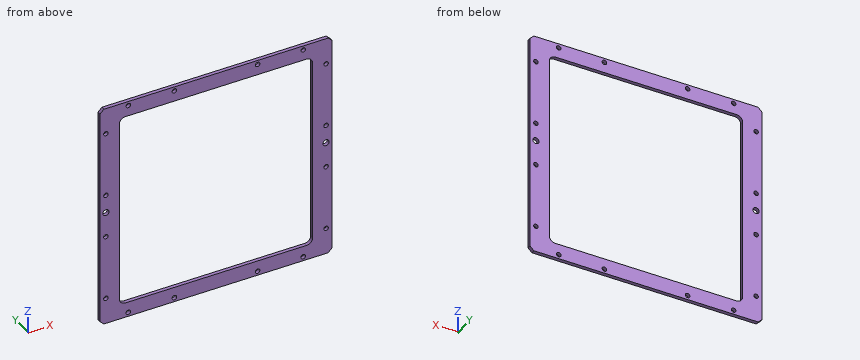
Autodesk Fusion 360 part; units mm, degrees
sketch "Front" plane through (0, 0, 0) normal (0, 1, 0) x (1, 0, 0) in component "1006350A"
  line L0 (-97.5923, -201.9946) -> (221.2351, -201.9946) construction
  line L1 (-99.947, -6.4146) -> (290.3014, -6.4146) construction
  line L2 (12.4997, 61.7326) -> (12.4997, -271.4585) construction
  line L3 (208.0797, 69.9741) -> (208.0797, -187.16) construction
  line L4 (213.4645, 13.4611) -> (213.4645, -265.3363) construction
  line L5 (7.1149, -256.6239) -> (7.1149, 6.397) construction
  line L6 (-10.9391, -2.6046) -> (257.2621, -2.6046) construction
  line L7 (3.4246, -205.8046) -> (275.1579, -205.8046) construction
  line L8 (196.1925, -231.664) -> (196.1925, 4.0423) construction
  line L9 (200.5105, 72.0933) -> (200.5105, -273.8132) construction
  line L10 (20.3229, -271.4585) -> (20.3229, 19.5833) construction
  line L11 (-9.5263, -26.3536) -> (218.174, -26.3536) construction
  line L12 (-30.2477, -84.6466) -> (216.2902, -84.6466) construction
  line L13 (226.8864, -107.3796) -> (-21.2998, -107.3796) construction
  line L14 (-47.6725, -123.7626) -> (220.7641, -123.7626) construction
  line L15 (-72.1615, -182.0556) -> (219.1158, -182.0556) construction
  line L16 (-7.1716, -192.3426) -> (237.718, -192.3426) construction
  line L17 (24.3869, -243.673) -> (24.3869, 8.2807) construction
  line L18 (187.7982, 11.5773) -> (187.7982, -213.2972) construction
  line L19 (147.2467, 23.5863) -> (147.2467, -210.9425) construction
  line L20 (73.3327, 36.3018) -> (73.3327, -224.8353) construction
  line L21 (32.4133, 51.8428) -> (32.4133, -217.3002) construction
  line L22 (267.4197, -11.8756) -> (2.5805, -11.8756) construction
  line L23 (267.0325, -196.4066) -> (1.4189, -196.4066) construction
  line L24 (1.5972, -16.0666) -> (220.1148, -16.0666) construction
  line L25 (7.1149, -205.8046) -> (213.4645, -205.8046)
  line L26 (213.4645, -205.8046) -> (213.4645, -2.6046)
  line L27 (213.4645, -2.6046) -> (7.1149, -2.6046)
  line L28 (7.1149, -2.6046) -> (7.1149, -205.8046)
  line L29 (24.3869, -192.3426) -> (196.1925, -192.3426)
  line L30 (196.1925, -192.3426) -> (196.1925, -16.0666)
  line L31 (196.1925, -16.0666) -> (24.3869, -16.0666)
  line L32 (24.3869, -16.0666) -> (24.3869, -192.3426)
  point P0 (32.4133, -201.9946)
  point P1 (73.3327, -201.9946)
  point P2 (147.2467, -201.9946)
  point P3 (187.7982, -201.9946)
  point P4 (208.0797, -182.0556)
  point P5 (208.0797, -123.7626)
  point P6 (208.0797, -107.3796)
  point P7 (208.0797, -84.6466)
  point P8 (208.0797, -26.3536)
  point P9 (187.7982, -6.4146)
  point P10 (147.2467, -6.4146)
  point P11 (73.3327, -6.4146)
  point P12 (32.4133, -6.4146)
  point P13 (12.4997, -26.3536)
  point P14 (12.4997, -84.6466)
  point P15 (12.4997, -107.3796)
  point P16 (12.4997, -123.7626)
  point P17 (12.4997, -182.0556)
  dimension "d1" = 195.58
  dimension "d2" = 3.81
  dimension "d3" = 19.939
  dimension "d4" = 78.232
  dimension "d5" = 117.348
  dimension "d6" = 175.641
  dimension "d7" = 100.965
  dimension "d10" = 5.3848
  dimension "d11" = 17.272
  dimension "d12" = 60.833
  dimension "d13" = 134.747
  dimension "d14" = 175.6664
  dimension "d15" = 195.58
  dimension "d16" = 203.2
  dimension "d17" = 184.531
  dimension "d18" = 5.461
  dimension "d19" = 13.462
  dimension "d20" = 189.0776
  dimension "d21" = 206.3496
  dimension "d22" = 13.462
  dimension "d33" = 7.5692
  dimension "d34" = 180.1876
extrude "Extrude1" add sketch "Front" along normal blind 3.175 in component "1006350A"
chamfer "Chamfer1" distance 3.556 angle 45 4 edges at (7.1149, 1.5875, 205.8046) (213.4645, 1.5875, 205.8046) (213.4645, 1.5875, 2.6046) (7.1149, 1.5875, 2.6046) in component "1006350A"
fillet "Fillet1" radius 5.5372 4 edges at (196.1925, 1.5875, 192.3426) (24.3869, 1.5875, 192.3426) (24.3869, 1.5875, 16.0666) (196.1925, 1.5875, 16.0666) in component "1006350A"
hole "Hole1" at (12.4997, 0, 107.3796) at (208.0797, 0, 107.3796) direction (0, 1, 0) diameter 5.5372 end through all in component "1006350A"
hole "Hole2" at (147.2467, 0, 201.9946) at (187.7982, 0, 201.9946) at (208.0797, 0, 182.0556) at (208.0797, 0, 123.7626) at (73.3327, 0, 201.9946) at (32.4133, 0, 201.9946) at (12.4997, 0, 182.0556) at (12.4997, 0, 123.7626) at (12.4997, 0, 84.6466) at (12.4997, 0, 26.3536) at (32.4133, 0, 6.4146) at (73.3327, 0, 6.4146) at (147.2467, 0, 6.4146) at (187.7982, 0, 6.4146) at (208.0797, 0, 26.3536) at (208.0797, 0, 84.6466) direction (0, 1, 0) diameter 4.0894 end through all in component "1006350A"
component "1006350A" placed x (1, 0, 0) y (0, 1, 0) z (0, 0, 1) at (0, 0, 0)
Work out the finished part from the listing and answer in its coordinate system (mm). Give positions to 0.01 mm unless a question says otherwise; leave off trailing zeros. Loops run counter-clockwise (first coordinate to the right, second up) from the corner with the lowest first, then second, coordinate; pieces in that order, holes last. Notation, with made-up numbers: (1, 10.25) - (23, 10.25) arc R30 cw to (23, 43.25) - close; hole circle Ø10 at (64.25, -22). An arc over 180 degrees is marked (long way). Answer in a Markdown table with one row per item.
(1) Section C-C (y = 1.45) is taken. State how many separate pieces and enclosed holes the cut face has, and give its area (3 significant figures).
Results list:
| item | result |
|---|---|
| separate pieces | 1 |
| enclosed holes | 19 |
| area | 11,400 mm² |
(2) Section A-A (z = 164.5) is taken. Give the vertices of the cut face in (x, y) (1 decimal).
Results list:
| item | result |
|---|---|
| outline | (7.1, 0) - (24.4, 0) - (24.4, 3.2) - (7.1, 3.2) - close; (196.2, 0) - (213.5, 0) - (213.5, 3.2) - (196.2, 3.2) - close |
(3) Consider L1, parallel to X at y = 1.8, z = 156; L2, parallel to Z at x = 149.5, y = 1.4; L3, parallel to X at y = 0.8, z = 187.5. Determine where each line is inside the solid, lowest interval first. Write a range as [from, to].
Results list:
| item | result |
|---|---|
| L1 | x = [7.11, 24.39], [196.19, 213.46] |
| L2 | z = [2.6, 16.07], [192.34, 205.8] |
| L3 | x = [7.11, 24.43], [196.15, 213.46] |
(4) Section B-B (x = 47) is taken. Give the vertices of the cut face in (y, z) (3 decimals).
Results list:
| item | result |
|---|---|
| outline | (0, 2.605) - (3.175, 2.605) - (3.175, 16.067) - (0, 16.067) - close; (0, 192.343) - (3.175, 192.343) - (3.175, 205.805) - (0, 205.805) - close |
